from build123d import *

# Parameters (mm, degrees)
SKETCH2_W           = 50
SKETCH2_H           = 50
SKETCH2_W_2         = 46
SKETCH2_H_2         = 46
SKETCH3_W           = 65
SKETCH3_H           = 50
BOSS_EXTRUDE1_DEPTH = 2
SKETCH4_W           = 50
SKETCH4_H           = 65
BOSS_EXTRUDE2_DEPTH = 2
SKETCH5_W           = 2
SKETCH5_H           = 65
SKETCH5_W_2         = 65
SKETCH5_H_2         = 2
BOSS_EXTRUDE3_DEPTH = 50
SKETCH6_W           = 65
SKETCH6_H           = 50
SKETCH6_W_2         = 50
SKETCH6_H_2         = 65
BOSS_EXTRUDE4_DEPTH = 48
SKETCH7_W           = 50
SKETCH7_H           = 65
SKETCH7_W_2         = 65
SKETCH7_H_2         = 50
CUT_EXTRUDE1_DEPTH  = 48


with BuildPart() as part:
    # Sweep1: sweep along a path in Sketch1
    with BuildLine(Plane.XY) as sweep1_path:
        Line((-615, 1265), (0, 1265))
        Line((0, 1265), (0, 0))
    # Sketch2 → Sweep1 (sweep)
    with BuildSketch(Plane(origin=(0, 0, 0), x_dir=(1, 0, 0), z_dir=(0, 1, 0))):
        with Locations((-25, 0)):
            Rectangle(SKETCH2_W, SKETCH2_H)
        with Locations((-25, 0)):
            Rectangle(SKETCH2_W_2, SKETCH2_H_2, mode=Mode.SUBTRACT)
    sweep(path=sweep1_path.line, transition=Transition.RIGHT)

    # Sketch3 → Boss-Extrude1 (add)
    with BuildSketch(Plane.XY.offset(25)):
        with Locations((-25, -25)):
            Rectangle(SKETCH3_W, SKETCH3_H)
    extrude(amount=-BOSS_EXTRUDE1_DEPTH)

    # Sketch4 → Boss-Extrude2 (add)
    with BuildSketch(Plane.XY.offset(25)):
        with Locations((-640, 1240)):
            Rectangle(SKETCH4_W, SKETCH4_H)
    extrude(amount=-BOSS_EXTRUDE2_DEPTH)

    # Sketch5 → Boss-Extrude3 (add)
    with BuildSketch(Plane.XY.offset(25)):
        with Locations((-614, 1240)):
            Rectangle(SKETCH5_W, SKETCH5_H)
        with Locations((-25, 1)):
            Rectangle(SKETCH5_W_2, SKETCH5_H_2)
    extrude(amount=-BOSS_EXTRUDE3_DEPTH)

    # Sketch6 → Boss-Extrude4 (add)
    with BuildSketch(Plane(origin=(0, 0, 23), x_dir=(-1, 0, 0), z_dir=(0, 0, -1))):
        with Locations((25, -25)):
            Rectangle(SKETCH6_W, SKETCH6_H)
        with Locations((640, 1240)):
            Rectangle(SKETCH6_W_2, SKETCH6_H_2)
    extrude(amount=BOSS_EXTRUDE4_DEPTH)

    # Sketch7 → Cut-Extrude1 (cut)
    with BuildSketch(Plane.XY.offset(25)):
        with Locations((-640, 1240)):
            Rectangle(SKETCH7_W, SKETCH7_H)
        with Locations((-25, -25)):
            Rectangle(SKETCH7_W_2, SKETCH7_H_2)
    extrude(amount=-CUT_EXTRUDE1_DEPTH, mode=Mode.SUBTRACT)


solid = part.part
For this review, take the finished solid that the model builds, in its own axes (mm). A direction names the side the tool comes from. Round coordinates to 2 decimals unless told otherwise and drop trailing zeros. Write each loop counter-clockwise with the first axis right and the second up, starting at its lowest first coordinate (ties: lowest second). Pieces come first, ordered by that corner, then holes. Notation, with made-up numbers: (4, 26) -> (41, 26) arc R6 cw to (41, 37) -> close; hole circle Ø6 at (18, 43). An arc over 180 degrees is marked (long way). Put each result on its own line as item: value.
Q1. Consider section A-A on y = 95.5. State the section outline as (x, z) points, and give its area (3 significant figures).
Determined:
outline: (-50, -25) -> (0, -25) -> (0, 25) -> (-50, 25) -> close; hole (-48, -23) -> (-2, -23) -> (-2, 23) -> (-48, 23) -> close
area: 384 mm^2
Q2. Consider section C-C on x = -168. State the section outline as (y, z) points, and give its area (3 significant figures).
Determined:
outline: (1215, -25) -> (1265, -25) -> (1265, 25) -> (1215, 25) -> close; hole (1217, -23) -> (1263, -23) -> (1263, 23) -> (1217, 23) -> close
area: 384 mm^2
Q3. Machinability: for faces 5 (the flat face through (-25, -25, -23)), 6 (the flat face through (-628, 1207.5, -24)), 7 (the flat face through (-48, 601, 0)), which of the approach directions +Z, -Z, +X, -X, +Y, -Y give a long, thin tool a straight path to every point of the face, cutting with its end or side? Answer none if there is none.
Determined:
face 5: +Z, +X, -X, -Y
face 6: +Z, -Z, -X, -Y
face 7: none
Q4. Consider section B-B on z = -5. State the section outline as (x, y) points.
Determined:
outline: (-615, 1207.5) -> (-613, 1207.5) -> (-613, 1215) -> (-50, 1215) -> (-50, 2) -> (-57.5, 2) -> (-57.5, 0) -> (7.5, 0) -> (7.5, 2) -> (0, 2) -> (0, 1265) -> (-613, 1265) -> (-613, 1272.5) -> (-615, 1272.5) -> close; hole (-613, 1217) -> (-48, 1217) -> (-48, 2) -> (-2, 2) -> (-2, 1263) -> (-613, 1263) -> close
Q5. To check wall thickness, follow L1, parallel to Y at x = -315, z = -2.5; L2, parallel to X at y = 874, z = -3; L3, parallel to Y at x = -39.5, z = -12. State the ranges of each line that lie inside material, in increasing order. Write a range as [from, to].
Determined:
L1: y = [1215, 1217], [1263, 1265]
L2: x = [-50, -48], [-2, 0]
L3: y = [0, 2], [1263, 1265]
Q6. Clearance check with flat-ended pins moving along their axes: pin 1 Ø23 at (x, z) = (-221, -9) entering from +Y; pin 2 Ø25 at (x, z) = (-326, 7.5) entering from -Y; pin 3 Ø5 at (y, z) = (733.5, -3.5) entering from +X. State where each tip first meets the part, or that it passes through.
Determined:
pin 1: stops at y = 1265
pin 2: stops at y = 1215
pin 3: stops at x = 0
Q7. Consider section D-D on x = -35.5. State the section outline as (y, z) points, and give its area (3 significant figures).
Determined:
outline: (-50, -25) -> (1265, -25) -> (1265, 25) -> (0, 25) -> (0, -23) -> (-50, -23) -> close; hole (2, -23) -> (1263, -23) -> (1263, 23) -> (2, 23) -> close
area: 5,340 mm^2
Q8. The part is to be moulded in two halves that separate along Z. For faces 1 (the flat face through (-613, 1240, 0)), 2 (the flat face through (-640, 1240, -23)), 3 (the flat face through (-327, 1217, 0)), 4 (the flat face through (-50, 600, 0)), say which applies: released by +Z, released by -Z, zero draft, split by the parting line, or undercut.
Determined:
face 1: undercut
face 2: released by +Z
face 3: undercut
face 4: zero draft
